CAD build for the part. Positions are in the model's coordinates, mm. Round coordinates to 2 decimals unless told otherwise and drop trailing zeros. Loops run counter-clockwise (first coordinate to the right, second up) from the corner with the lowest first, then second, coordinate; pieces in that order, holes last. Notation, with made-up numbers: (65.25, 16.5) - (70.25, 16.5) arc R11 ccw to (70.25, 36.5) - close; hole circle Ø2 at (16, 50.25). An arc over 180 degrees is marked (long way). Use one line per item in the form item = value.
from build123d import *

# Parameters (mm, degrees)
SKETCH1_R           = 7.112
SKETCH1_R_2         = 2.54
SKETCH1_R_3         = 19.304
BOSS_EXTRUDE1_DEPTH = 3.302


with BuildPart() as part:
    # Sketch1 → Boss-Extrude1 (new body)
    with BuildSketch(Plane.XY):
        with BuildLine():
            Line((-38.1, 0), (-38.1, 88.9))
            Line((-38.1, 88.9), (38.1, 88.9))
            Line((38.1, 88.9), (38.1, 0))
            ThreePointArc((38.1, 0), (0, -38.1), (-38.1, 0))
        make_face()
        with Locations((23.57, 71.755)):
            Circle(SKETCH1_R, mode=Mode.SUBTRACT)
        with Locations((23.57, 23.495)):
            Circle(SKETCH1_R_2, mode=Mode.SUBTRACT)
        with Locations((-23.57, -23.495)):
            Circle(SKETCH1_R_2, mode=Mode.SUBTRACT)
        with Locations((-23.57, 23.495)):
            Circle(SKETCH1_R_2, mode=Mode.SUBTRACT)
        with Locations((-23.57, 71.755)):
            Circle(SKETCH1_R, mode=Mode.SUBTRACT)
        with Locations((23.57, -23.495)):
            Circle(SKETCH1_R_2, mode=Mode.SUBTRACT)
        Circle(SKETCH1_R_3, mode=Mode.SUBTRACT)
    extrude(amount=BOSS_EXTRUDE1_DEPTH)


solid = part.part
1) Slice it at B-B (y = 3). Write the cut outline in (x, z), plus the area to 3 significant figures.
Report:
outline = (-38.1, 0) - (-19.07, 0) - (-19.07, 3.3) - (-38.1, 3.3) - close; (19.07, 0) - (38.1, 0) - (38.1, 3.3) - (19.07, 3.3) - close
area = 126 mm^2
2) Two-plate mould, pull along Y, no slides. Class faces 1 (the cylindrical face through (0.84, -38.09, 1.63)), 2 (the cylindrical face through (21.032, -23.383, 1.628)), 3 (the flat face through (-38.1, 44, 2)): +Y half, -Y half, draft (parallel to the pull), parting line (faces both ways), or undercut.
Report:
face_1 = -Y half
face_2 = undercut
face_3 = draft
3) Slice it at A-A (x = 0). Write the cut outline in (y, z), plus the area to 3 significant figures.
Report:
outline = (-38.1, 0) - (-19.3, 0) - (-19.3, 3.3) - (-38.1, 3.3) - close; (19.3, 0) - (88.9, 0) - (88.9, 3.3) - (19.3, 3.3) - close
area = 292 mm^2
4) Flat gauge pins, fed straight in: pin 1 (12 mm diameter, centred on x = 13, y = 53.5, fed in from -Z); pin 2 (1 mm diameter, centred on x = 9, z = 2, fed in from -Y). Where does each tip first touch, or does it go through?
Report:
pin_1 = 0
pin_2 = -37.14
5) Drill centre lines: probe 1 along X at (y, z) = (72, 0.65); probe 2 along Y at (x, z) = (-23.57, 2.25) (3 decimals); probe 3 along Y at (x, z) = (0, 1.9). Where is each one in solid material? Low to high.
Report:
probe_1 = -38.1 to -30.68, -16.46 to 16.46, 30.68 to 38.1
probe_2 = -29.934 to -26.035, -20.955 to 20.955, 26.035 to 64.643, 78.867 to 88.9
probe_3 = -38.1 to -19.3, 19.3 to 88.9
6) Slice it at C-C (x = -23.57). Write the cut outline in (y, z) (3 decimals), plus the area to 3 significant figures.
Report:
outline = (-29.934, 0) - (-26.035, 0) - (-26.035, 3.302) - (-29.934, 3.302) - close; (-20.955, 0) - (20.955, 0) - (20.955, 3.302) - (-20.955, 3.302) - close; (26.035, 0) - (64.643, 0) - (64.643, 3.302) - (26.035, 3.302) - close; (78.867, 0) - (88.9, 0) - (88.9, 3.302) - (78.867, 3.302) - close
area = 312 mm^2
7) Slice it at D-D (z = 2.7). Write the cut outline in (x, y) (3 decimals).
Report:
outline = (-38.1, 0) arc R38.1 ccw to (38.1, 0) - (38.1, 88.9) - (-38.1, 88.9) - close; hole circle Ø14.224 at (-23.57, 71.755); hole circle Ø5.08 at (-23.57, -23.495); hole circle Ø5.08 at (-23.57, 23.495); hole circle Ø38.608 at (0, 0); hole circle Ø14.224 at (23.57, 71.755); hole circle Ø5.08 at (23.57, -23.495); hole circle Ø5.08 at (23.57, 23.495)
